Read the model definition and answer for the solid it produces. Units are mm, in the model's axes. Round coordinates to 2 decimals unless told otherwise and drop trailing zeros. Order: outer loops, then holes, each group sorted by start corner. A loop starts at its lowest first (then second) coordinate and runs counter-clockwise, first axis right, second up. Notation, with made-up numbers: (24, 21) - (56, 21) arc R38 ccw to (56, 59) - close; hole circle Ø10 at (24.5, 41). An arc over 180 degrees is marked (long way). Put each result on its own line as item: value. Start each with the question number.
Q1. Find the intervals of material crossed by line 1 along Z through (x, y) = (0, -0.9); line 2 along X through (y, z) = (-1.15, -10.5); line 3 along Z through (x, y) = (-13, -0.65), in increasing order. Write a range as from..to.
Q2. Each of these flat-tipped pins is pushed along its axis until it touches: pin 1 Ø1 at (y, z) = (-1, 17) entering from -X; pin 2 Ø1 at (y, z) = (-1, -6) entering from -X; pin 3 Ø1.5 at (x, z) = (-12, -13) entering from +Y; pin 4 Ø1 at (y, z) = (-1, -7) entering from +X. Where does it stop, or does it pass through?
Q3. Section B-B on z = 0 is taken. Give the vertices of the cut face in (x, y), then the cut area to 3 significant figures.
Q4. Section A-A on x = 0 is taken. Give the vertices of the cut face in (y, z), then the cut area to 3 significant figures.
from build123d import *

# Parameters (mm, degrees)
F0_R     = 3
F1_DEPTH = 2


with BuildPart() as f1:
    # F0 (on Front) → F1 (new body)
    with BuildSketch(Plane.XZ):
        with BuildLine():
            Line((-1, 10), (-1, 4.898979))
            ThreePointArc((-1, 4.898979), (-2.5, 4.330127), (-3.742641, 3.315515))
            Line((-3.742641, 3.315515), (-8.160254, 5.866025))
            Line((-8.160254, 5.866025), (-9.971987, 12.627506))
            ThreePointArc((-9.971987, 12.627506), (-11.196732, 13.334613), (-11.903839, 12.109868))
            Line((-11.903839, 12.109868), (-10.609744, 7.280239))
            Line((-10.609744, 7.280239), (-16.820508, 10.866025))
            ThreePointArc((-16.820508, 10.866025), (-18.186533, 10.5), (-17.820508, 9.133975))
            Line((-17.820508, 9.133975), (-11.609744, 5.548188))
            Line((-11.609744, 5.548188), (-16.439373, 4.254093))
            ThreePointArc((-16.439373, 4.254093), (-17.14648, 3.029348), (-15.921735, 2.322241))
            Line((-15.921735, 2.322241), (-9.160254, 4.133975))
            Line((-9.160254, 4.133975), (-4.742641, 1.583464))
            ThreePointArc((-4.742641, 1.583464), (-5, 0), (-4.742641, -1.583464))
            Line((-4.742641, -1.583464), (-9.160254, -4.133975))
            Line((-9.160254, -4.133975), (-15.921735, -2.322241))
            ThreePointArc((-15.921735, -2.322241), (-17.14648, -3.029348), (-16.439373, -4.254093))
            Line((-16.439373, -4.254093), (-11.609744, -5.548188))
            Line((-11.609744, -5.548188), (-17.820508, -9.133975))
            ThreePointArc((-17.820508, -9.133975), (-18.186533, -10.5), (-16.820508, -10.866025))
            Line((-16.820508, -10.866025), (-10.609744, -7.280239))
            Line((-10.609744, -7.280239), (-11.903839, -12.109868))
            ThreePointArc((-11.903839, -12.109868), (-11.196732, -13.334613), (-9.971987, -12.627506))
            Line((-9.971987, -12.627506), (-8.160254, -5.866025))
            Line((-8.160254, -5.866025), (-3.742641, -3.315515))
            ThreePointArc((-3.742641, -3.315515), (-2.5, -4.330127), (-1, -4.898979))
            Line((-1, -4.898979), (-1, -10))
            Line((-1, -10), (-5.949747, -14.949747))
            ThreePointArc((-5.949747, -14.949747), (-5.949747, -16.363961), (-4.535534, -16.363961))
            Line((-4.535534, -16.363961), (-1, -12.828427))
            Line((-1, -12.828427), (-1, -20))
            ThreePointArc((-1, -20), (0, -21), (1, -20))
            Line((1, -20), (1, -12.828427))
            Line((1, -12.828427), (4.535534, -16.363961))
            ThreePointArc((4.535534, -16.363961), (5.949747, -16.363961), (5.949747, -14.949747))
            Line((5.949747, -14.949747), (1, -10))
            Line((1, -10), (1, -4.898979))
            ThreePointArc((1, -4.898979), (2.5, -4.330127), (3.742641, -3.315515))
            Line((3.742641, -3.315515), (8.160254, -5.866025))
            Line((8.160254, -5.866025), (9.971987, -12.627506))
            ThreePointArc((9.971987, -12.627506), (11.196732, -13.334613), (11.903839, -12.109868))
            Line((11.903839, -12.109868), (10.609744, -7.280239))
            Line((10.609744, -7.280239), (16.820508, -10.866025))
            ThreePointArc((16.820508, -10.866025), (18.186533, -10.5), (17.820508, -9.133975))
            Line((17.820508, -9.133975), (11.609744, -5.548188))
            Line((11.609744, -5.548188), (16.439373, -4.254093))
            ThreePointArc((16.439373, -4.254093), (17.14648, -3.029348), (15.921735, -2.322241))
            Line((15.921735, -2.322241), (9.160254, -4.133975))
            Line((9.160254, -4.133975), (4.742641, -1.583464))
            ThreePointArc((4.742641, -1.583464), (5, 0), (4.742641, 1.583464))
            Line((4.742641, 1.583464), (9.160254, 4.133975))
            Line((9.160254, 4.133975), (15.921735, 2.322241))
            ThreePointArc((15.921735, 2.322241), (17.14648, 3.029348), (16.439373, 4.254093))
            Line((16.439373, 4.254093), (11.609744, 5.548188))
            Line((11.609744, 5.548188), (17.820508, 9.133975))
            ThreePointArc((17.820508, 9.133975), (18.186533, 10.5), (16.820508, 10.866025))
            Line((16.820508, 10.866025), (10.609744, 7.280239))
            Line((10.609744, 7.280239), (11.903839, 12.109868))
            ThreePointArc((11.903839, 12.109868), (11.196732, 13.334613), (9.971987, 12.627506))
            Line((9.971987, 12.627506), (8.160254, 5.866025))
            Line((8.160254, 5.866025), (3.742641, 3.315515))
            ThreePointArc((3.742641, 3.315515), (2.5, 4.330127), (1, 4.898979))
            Line((1, 4.898979), (1, 10))
            Line((1, 10), (5.949747, 14.949747))
            ThreePointArc((5.949747, 14.949747), (5.949747, 16.363961), (4.535534, 16.363961))
            Line((4.535534, 16.363961), (1, 12.828427))
            Line((1, 12.828427), (1, 20))
            ThreePointArc((1, 20), (0, 21), (-1, 20))
            Line((-1, 20), (-1, 12.828427))
            Line((-1, 12.828427), (-4.535534, 16.363961))
            ThreePointArc((-4.535534, 16.363961), (-5.949747, 16.363961), (-5.949747, 14.949747))
            Line((-5.949747, 14.949747), (-1, 10))
        make_face()
        Circle(F0_R, mode=Mode.SUBTRACT)
    extrude(amount=F1_DEPTH)


solid = f1.part
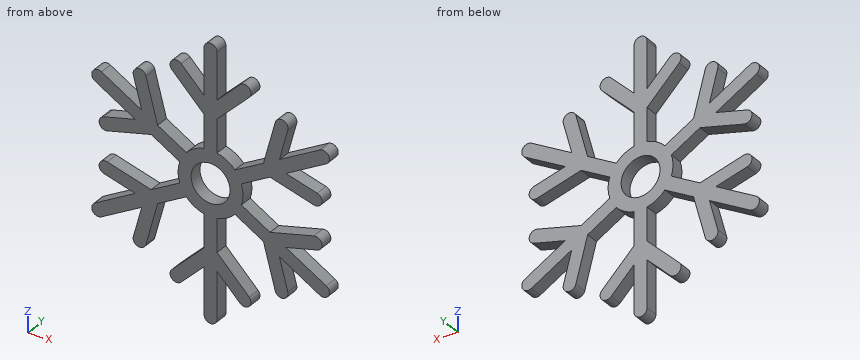
Findings:
1. line 1: -21..-3, 3..21
1. line 2: -18.19..-16.19, -11.47..-9.4, -1.5..1.5, 9.4..11.47, 16.19..18.19
1. line 3: -8.66..-6.35, -5.18..-3.11, 3.11..5.18, 6.35..8.66
2. pin 1: x = -5.78
2. pin 2: x = -13.26
2. pin 3: y = 0
2. pin 4: x = 14.99
3. outline: (-5, -2) - (-3, -2) - (-3, 0) - (-5, 0) - close; (3, -2) - (5, -2) - (5, 0) - (3, 0) - close
3. area: 8.00 mm2
4. outline: (-2, -21) - (0, -21) - (0, -3) - (-2, -3) - close; (-2, 3) - (0, 3) - (0, 21) - (-2, 21) - close
4. area: 72.0 mm2
